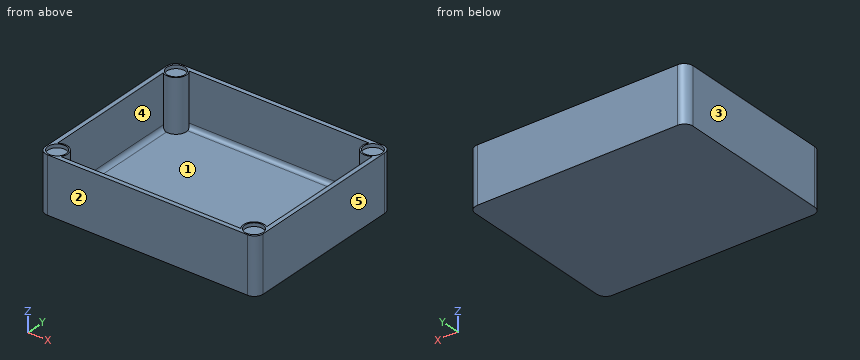
from build123d import *

# Parameters (mm, degrees)
SKETCH_W        = 125
SKETCH_H        = 100
PAD_DEPTH       = 32
SKETCH001_W     = 120
SKETCH001_H     = 95
POCKET_DEPTH    = 32
SKETCH002_R     = 6
PAD001_DEPTH    = 30
SKETCH003_R     = 5.25
POCKET001_DEPTH = 2
FILLET_R        = 2.5
FILLET001_R     = 2.5
FILLET002_R     = 2.5
FILLET003_R     = 2.5
FILLET004_R     = 5
FILLET005_R     = 5
FILLET006_R     = 5
FILLET007_R     = 5


with BuildPart() as part:
    # Sketch → Pad (new body)
    with BuildSketch(Plane.XY):
        with Locations((62.5, 50)):
            Rectangle(SKETCH_W, SKETCH_H)
    extrude(amount=PAD_DEPTH)

    # Sketch001 → Pocket (cut)
    with BuildSketch(Plane.XY.offset(34)):
        with Locations((62.5, 50)):
            Rectangle(SKETCH001_W, SKETCH001_H)
    extrude(amount=-POCKET_DEPTH, mode=Mode.SUBTRACT)

    # Sketch002 (on Face11 of Pocket) → Pad001 (join)
    with BuildSketch(Plane.XY.offset(2)):
        with Locations((6, 6)):
            Circle(SKETCH002_R)
        with Locations((6, 94)):
            Circle(SKETCH002_R)
        with Locations((119, 94)):
            Circle(SKETCH002_R)
        with Locations((119, 6)):
            Circle(SKETCH002_R)
    extrude(amount=PAD001_DEPTH)

    # Sketch003 (on Face27 of Pad001) → Pocket001 (cut)
    with BuildSketch(Plane.XY.offset(32)):
        with Locations((6, 6)):
            Circle(SKETCH003_R)
        with Locations((6, 94)):
            Circle(SKETCH003_R)
        with Locations((119, 94)):
            Circle(SKETCH003_R)
        with Locations((119, 6)):
            Circle(SKETCH003_R)
    extrude(amount=-POCKET001_DEPTH, mode=Mode.SUBTRACT)

    # Fillet
    fillet_edges = [part.edges().sort_by_distance(p)[0] for p in [
        (62.5, 2.5, 2),
    ]]
    fillet(fillet_edges, radius=FILLET_R)

    # Fillet001
    fillet001_edges = [part.edges().sort_by_distance(p)[0] for p in [
        (122.5, 50, 2),
    ]]
    fillet(fillet001_edges, radius=FILLET001_R)

    # Fillet002
    fillet002_edges = [part.edges().sort_by_distance(p)[0] for p in [
        (62.5, 97.5, 2),
    ]]
    fillet(fillet002_edges, radius=FILLET002_R)

    # Fillet003
    fillet003_edges = [part.edges().sort_by_distance(p)[0] for p in [
        (2.5, 50, 2),
    ]]
    fillet(fillet003_edges, radius=FILLET003_R)

    # Fillet004
    fillet004_edges = [part.edges().sort_by_distance(p)[0] for p in [
        (125, 100, 16),
    ]]
    fillet(fillet004_edges, radius=FILLET004_R)

    # Fillet005
    fillet005_edges = [part.edges().sort_by_distance(p)[0] for p in [
        (125, 0, 16),
    ]]
    fillet(fillet005_edges, radius=FILLET005_R)

    # Fillet006
    fillet006_edges = [part.edges().sort_by_distance(p)[0] for p in [
        (0, 0, 16),
    ]]
    fillet(fillet006_edges, radius=FILLET006_R)

    # Fillet007
    fillet007_edges = [part.edges().sort_by_distance(p)[0] for p in [
        (0, 100, 16),
    ]]
    fillet(fillet007_edges, radius=FILLET007_R)


solid = part.part
For this review, take the finished solid that the model builds, in its own axes (mm). Face numbers are marked on the shaded views. A direction names the side the tool comes from. Round coordinates to 2 decimals unless told otherwise and drop trailing zeros. Order: outer loops, then holes, each group sorted by start corner. A loop starts at its lowest first (then second) coordinate and runs counter-clockwise, first axis right, second up. Notation, with made-up numbers: (-24.5, 60) -> (-10.5, 60) arc R27 ccw to (-10.5, 87) -> close; hole circle Ø1 at (43, 84.5). An arc over 180 degrees is marked (long way). Put each result on its own line as item: value.
Q1. Machinability: for the marked faces 4 and 5, which of the approach directions +Z, -Z, +X, -X, +Y, -Y give a long, thin tool a straight path to every point of the face, cutting with its end or side? Answer none if there is none.
Check result:
face 4: +Z
face 5: +Z, -Z, +X, +Y, -Y
Q2. Add section B-B on z = 18. Write out the cut boundary in (x, y).
Check result:
outline: (0, 5) arc R5 ccw to (5, 0) -> (120, 0) arc R5 ccw to (125, 5) -> (125, 95) arc R5 ccw to (120, 100) -> (5, 100) arc R5 ccw to (0, 95) -> close; hole (2.5, 10.87) arc R6 cw to (10.87, 2.5) -> (114.13, 2.5) arc R6 cw to (122.5, 10.87) -> (122.5, 89.13) arc R6 cw to (114.13, 97.5) -> (10.87, 97.5) arc R6 cw to (2.5, 89.13) -> close
Q3. Mouldability with a two-part tool opening along Y and no side actions: class the marked faces 1, 2 and 3 as pulls with the +Y half, pulls with the -Y half, needs draft (parallel to the pull), parting line crosses it, or undercut.
Check result:
face 1: undercut
face 2: pulls with the -Y half
face 3: needs draft
Q4. Add section C-C on x = 102. Write out the cut boundary in (y, z), plus the area to 3 significant figures.
Check result:
outline: (0, 0) -> (100, 0) -> (100, 32) -> (97.5, 32) -> (97.5, 4.5) arc R2.5 cw to (95, 2) -> (5, 2) arc R2.5 cw to (2.5, 4.5) -> (2.5, 32) -> (0, 32) -> close
area: 353 mm2
Q5. For probe 1 along Y at (x, z) = (6, 31.55); probe 2 along X at (y, z) = (82, 14.5); probe 3 along Y at (x, z) = (102, 17.5), list the stretches that pass through material, from the lowest coordinate up. Write a range as [from, to].
Check result:
probe 1: [0, 0.75], [11.25, 12], [88, 88.75], [99.25, 100]
probe 2: [0, 2.5], [122.5, 125]
probe 3: [0, 2.5], [97.5, 100]
Q6. Insertion check: pin 1 Ø9.5 at (x, y) = (119, 6) entering from +Z; pin 2 Ø8.5 at (x, y) = (7.5, 91.5) entering from +Z; pin 3 Ø4 at (x, y) = (98.5, 83) entering from +Z. Each pin has a flat end and moves straight along its axis. Give the tip position at first contact, or say it passes through.
Check result:
pin 1: z = 30
pin 2: z = 32
pin 3: z = 2
Q7. Add section A-A on y = 45.5. Write out the cut boundary in (x, z), plus the area to 3 significant figures.
Check result:
outline: (0, 0) -> (125, 0) -> (125, 32) -> (122.5, 32) -> (122.5, 4.5) arc R2.5 cw to (120, 2) -> (5, 2) arc R2.5 cw to (2.5, 4.5) -> (2.5, 32) -> (0, 32) -> close
area: 403 mm2
